```python
from build123d import *

# Parameters (mm, degrees)
SKETCH_1_W          = 38
SKETCH_1_H          = 13
EXTRUDE_1_DEPTH     = 25
SKETCH_2_W          = 50.27368421
SKETCH_2_H          = 9
CUT_EXTRUDE_1_DEPTH = 15
SKETCH_3_W          = 20
SKETCH_3_H          = 30
CUT_EXTRUDE_2_DEPTH = 34.985290936
SKETCH_4_R          = 2.5
CUT_EXTRUDE_3_DEPTH = 34.985290936
SKETCH_8_R          = 2.5
EXTRUDE_3_DEPTH     = 7.5
SKETCH_9_W          = 5
SKETCH_9_H          = 54.936954578
CUT_EXTRUDE_5_DEPTH = 34.985290936


with BuildPart() as part:
    # 草图1 → 凸台-拉伸1 (new body)
    with BuildSketch(Plane.XY):
        Rectangle(SKETCH_1_W, SKETCH_1_H)
    extrude(amount=EXTRUDE_1_DEPTH)

    # 草图2 → 切除-拉伸1 (cut)
    with BuildSketch(Plane.XY.offset(25)):
        Rectangle(SKETCH_2_W, SKETCH_2_H)
    extrude(amount=-CUT_EXTRUDE_1_DEPTH, mode=Mode.SUBTRACT)

    # 草图3 → 切除-拉伸2 (cut, through all)
    with BuildSketch(Plane(origin=(0, 6.5, 0), x_dir=(1, 0, 0), z_dir=(0, 1, 0))):
        with Locations((0, -25)):
            Rectangle(SKETCH_3_W, SKETCH_3_H)
    extrude(amount=-CUT_EXTRUDE_2_DEPTH, mode=Mode.SUBTRACT)

    # 草图4 → 切除-拉伸3 (cut, through all)
    with BuildSketch(Plane(origin=(0, 6.5, 0), x_dir=(1, 0, 0), z_dir=(0, 1, 0))):
        with Locations(Location((-15, -17.5, 0), (0, 0, 270))):
            Circle(SKETCH_4_R)
        with Locations((15, -17.5)):
            Circle(SKETCH_4_R)
    extrude(amount=-CUT_EXTRUDE_3_DEPTH, mode=Mode.SUBTRACT)

    # 草图8 → 凸台-拉伸3 (add, symmetric)
    with BuildSketch(Plane(origin=(0, 0, 0), x_dir=(0, 0, -1), z_dir=(1, 0, 0))):
        with BuildLine():
            Line((15, -6.5), (0, -6.5))
            Line((0, -6.5), (0, 6.5))
            Line((0, 6.5), (15, 6.5))
            ThreePointArc((15, 6.5), (21.5, 0), (15, -6.5))
        make_face()
        with Locations((15, 0)):
            Circle(SKETCH_8_R, mode=Mode.SUBTRACT)
    extrude(amount=EXTRUDE_3_DEPTH, both=True)

    # 草图9 → 切除-拉伸5 (cut, through all)
    with BuildSketch(Plane(origin=(0, 6.5, 0), x_dir=(1, 0, 0), z_dir=(0, 1, 0))):
        with Locations((0, 27.468477289)):
            Rectangle(SKETCH_9_W, SKETCH_9_H)
    extrude(amount=-CUT_EXTRUDE_5_DEPTH, mode=Mode.SUBTRACT)


solid = part.part
```
Work out the finished part from the listing and answer in its coordinate system (mm). A direction names the side the tool comes from. Give positions to 0.01 mm unless a question says otherwise; leave off trailing zeros. Write each loop counter-clockwise with the first axis right and the second up, starting at its lowest first coordinate (ties: lowest second). Pieces come first, ordered by that corner, then holes.
(1) Which of the six approach directions +Z, -Z, +X, -X, +Y, -Y give full straight-line access (tool end or side, diameter ignored) to faces 4 (the flat face through (-7.5, 0, -11)), 5 (the flat face through (10, -5, 18)), 6 (the flat face through (-12.6, 4.5, 19.3)), 7 (the flat face through (0, 0, 0))?
Final values:
face 4: -Z, -X, +Y, -Y
face 5: +Z, +Y, -Y
face 6: +Z, +X, -X
face 7: -Z, +Y, -Y
(2) The mould has two halves that part along Y. Classify faces 1 (the cylindrical face through (5, 0.1, -21.5)), 2 (the flat face through (19, 0, 7)), 3 (the flat face through (-12.6, -4.5, 19.3)): pulls with the +Y half, pulls with the -Y half, needs draft (parallel to the pull), parting line crosses it, or undercut.
Final values:
face 1: parting line crosses it
face 2: needs draft
face 3: undercut
(3) The part is cut by section C-C on x = 15. Write down the section's boundary in (y, z), plus the area to 3 significant figures.
Final values:
outline: (-6.5, 0) - (6.5, 0) - (6.5, 15) - (4.5, 15) - (4.5, 10) - (-4.5, 10) - (-4.5, 15) - (-6.5, 15) - close; (-6.5, 20) - (-4.5, 20) - (-4.5, 25) - (-6.5, 25) - close; (4.5, 20) - (6.5, 20) - (6.5, 25) - (4.5, 25) - close
area: 170 mm2
(4) The part is cut by section B-B on z = 17.5. Count the separate pieces of the cut face and the enclosed holes in it, plus the area to 3 significant figures.
Final values:
separate pieces: 8
enclosed holes: 0
area: 32.0 mm2
(5) Straight lines are drawn through the part: line 1 (X direction, y = 5.55, z = 17.5); line 2 (X direction, y = 2.5, z = -4); line 3 (Z direction, x = 15, y = -4.95). For each, find the intervals that lie inside material, in ascending order.
Final values:
line 1: x = -19 to -17.5, -12.5 to -10, 10 to 12.5, 17.5 to 19
line 2: x = -7.5 to -2.5, 2.5 to 7.5
line 3: z = 0 to 15, 20 to 25
(6) The part is cut by section D-D on y = 5.25. Write down the section's boundary in (x, z).
Final values:
outline: (-19, 0) - (-7.5, 0) - (-7.5, -18.83) - (-2.5, -18.83) - (-2.5, 0) - (2.5, 0) - (2.5, -18.83) - (7.5, -18.83) - (7.5, 0) - (19, 0) - (19, 25) - (10, 25) - (10, 10) - (-10, 10) - (-10, 25) - (-19, 25) - close; hole circle Ø5 at (-15, 17.5); hole circle Ø5 at (15, 17.5)
(7) Flat-ended cylindrical pins translate along their axes: pin 1 Ø3 at (x, y) = (9, 0.5) entering from +Z; pin 2 Ø6.5 at (y, z) = (0, -15) entering from -X; pin 3 Ø4 at (y, z) = (-2.5, -10.5) entering from +X. Find the tip coordinate at first contact, or state that the pin passes through.
Final values:
pin 1: stops at z = 10
pin 2: stops at x = -7.5
pin 3: stops at x = 7.5
(8) The part is cut by section A-A on y = 0. Write down the section's boundary in (x, z), plus the area to 3 significant figures.
Final values:
outline: (-19, 0) - (-7.5, 0) - (-7.5, -12.5) - (-2.5, -12.5) - (-2.5, 0) - (2.5, 0) - (2.5, -12.5) - (7.5, -12.5) - (7.5, 0) - (19, 0) - (19, 10) - (-19, 10) - close; (-7.5, -21.5) - (-2.5, -21.5) - (-2.5, -17.5) - (-7.5, -17.5) - close; (2.5, -21.5) - (7.5, -21.5) - (7.5, -17.5) - (2.5, -17.5) - close
area: 545 mm2
